Part model, mm, in its own coordinate system. Face numbers are marked on the shaded views. A direction names the side the tool comes from. Coordinates: 2 decimals unless noted, no trailing zeros. Order: outer loops, then holes, each group sorted by start corner. A loop starts at its lowest first (then second) coordinate and runs counter-clockwise, first axis right, second up. Notation, with made-up numbers: M 54,-34.75 L 66,-34.75 A23 cw 66,-8.75 Z; hole C 68,-3 d3. An arc over 180 degrees is marked long. Write item = value, one per line. Start each with the question number.
from build123d import *

# Parameters (mm, degrees)
CROQUIS1_R              = 6
CROQUIS1_R_2            = 4
SALIENTE_EXTRUIR1_DEPTH = 20
CROQUIS2_R              = 6
SALIENTE_EXTRUIR2_DEPTH = 2
SALIENTE_EXTRUIR3_REACH = 25.58


with BuildPart() as part:
    # Croquis1 → Saliente-Extruir1 (new body)
    with BuildSketch(Plane.XY):
        Circle(CROQUIS1_R)
        Circle(CROQUIS1_R_2, mode=Mode.SUBTRACT)
    extrude(amount=SALIENTE_EXTRUIR1_DEPTH)

    # Croquis2 → Saliente-Extruir2 (add)
    with BuildSketch(Plane.XY.offset(20)):
        Circle(CROQUIS2_R)
    extrude(amount=SALIENTE_EXTRUIR2_DEPTH)

    # Saliente-Extruir3: up to this face of the body (flat: up to its plane)
    saliente_extruir3_end = Plane(part.part.faces().sort_by_distance((0, 0, 22))[0])
    # Croquis3 → Saliente-Extruir3 (add, up to the picked face)
    with BuildSketch(Plane(origin=(0, 0, 0), x_dir=(-1, 0, 0), z_dir=(0, 0, -1)), mode=Mode.PRIVATE) as saliente_extruir3_sk1:
        Polygon((-0.21844428, 21.994030808), (-3.21844428, 21.994030808), (-3.21844428, 3.994030808), (2.78155572, 3.994030808), (2.78155572, 21.994030808), align=None)
    saliente_extruir3_tool1 = split(extrude(saliente_extruir3_sk1.sketch, amount=-SALIENTE_EXTRUIR3_REACH, mode=Mode.PRIVATE), bisect_by=saliente_extruir3_end, keep=Keep.BOTH, mode=Mode.PRIVATE)
    add(saliente_extruir3_tool1.solids().sort_by(Axis((0.218444, 12.994031, 0), (0, 0, 1)))[0])


solid = part.part
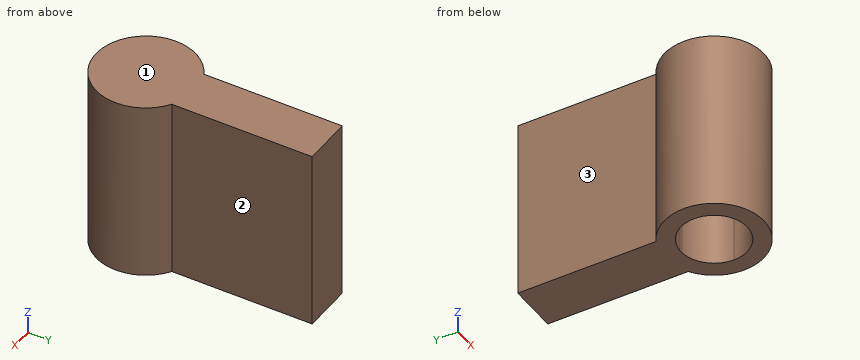
Item 1: 3-axis set-ups, long thin cutter, end or side, ignore diameter. For the marked faces 1, 2 and 3: which of +Z, -Z, +X, -X, +Y, -Y reach the whole face in a straight line?
Item 2: Cut at B-B, the plane x = -2.25. Write the cut outline in (y, z), and give its area (3 significant figures).
Item 3: Flat gauge pins, fed straight in: pin 1 (3 mm diameter, centred on y = 6, z = 13, fed in from -X); pin 2 (6 mm diameter, centred on y = 18.5, z = 7, fed in from -X); pin 3 (1 mm diameter, centred on x = 1.5, z = 19, fed in from -Y). Where does each tip first touch, or does it go through?
Item 4: Cut at A-A, the plane z = 9.75. Write the cut outline in (x, y), and give its area (3 significant figures).
Item 5: Wall check: line 1 along X through (y, z) = (0, 6.5); line 2 along X through (y, z) = (7, 9.75); line 3 along Y through (x, z) = (0, 5.5). Give the ranges that are in metal, low to high. Write a range as [from, to].
Item 6: Cut at D-D, the plane x = 2. Write the cut outline in (y, z).
Item 7: Cut at C-C, the plane y = 8.25. Write the cut outline in (x, z).
Filled sheet:
q1.face_1 = +Z, +X, -X, +Y, -Y
q1.face_2 = +Z, -Z, +X, +Y
q1.face_3 = +Z, -Z, -X, +Y
q2.outline = M -5.56,0 L -3.31,0 L -3.31,20 L 3.31,20 L 3.31,0 L 21.99,0 L 21.99,22 L -5.56,22 Z
q2.area = 474 mm2
q3.pin_1 = -3.97
q3.pin_2 = -2.78
q3.pin_3 = -5.92
q4.outline = M -2.78,5.32 A6 ccw long 3.22,5.06 L 3.22,21.99 L -2.78,21.99 Z; hole M -0.22,3.99 A4 ccw long 0.22,3.99 Z
q4.area = 160 mm2
q5.line_1 = [-6, -4], [4, 6]
q5.line_2 = [-2.78, 3.22]
q5.line_3 = [-6, -4], [3.99, 21.99]
q6.outline = M -5.66,0 L -3.46,0 L -3.46,20 L 3.46,20 L 3.46,0 L 21.99,0 L 21.99,22 L -5.66,22 Z
q7.outline = M -2.78,0 L 3.22,0 L 3.22,22 L -2.78,22 Z
